Input: dimensioned drawing with shaded views. Units: mm. Origin: part minimum x, y, z. Give positions to 0.01 mm unless a question says otherwise; leave off trailing zeros. Write each loop counter-clockwise with the first axis right and the second up, starting at its lowest first coordinate (ties: lowest second). Pieces come first, ordered by that corner, then holes. Notation, with made-up numbers: (57.5, 14) - (79.5, 14) arc R25 ccw to (79.5, 46) - close; hole circle Ø8 at (35.25, -13.75). An arc over 180 degrees is marked (long way). Answer as a JSON object with one key per item and string values. Group by question number.
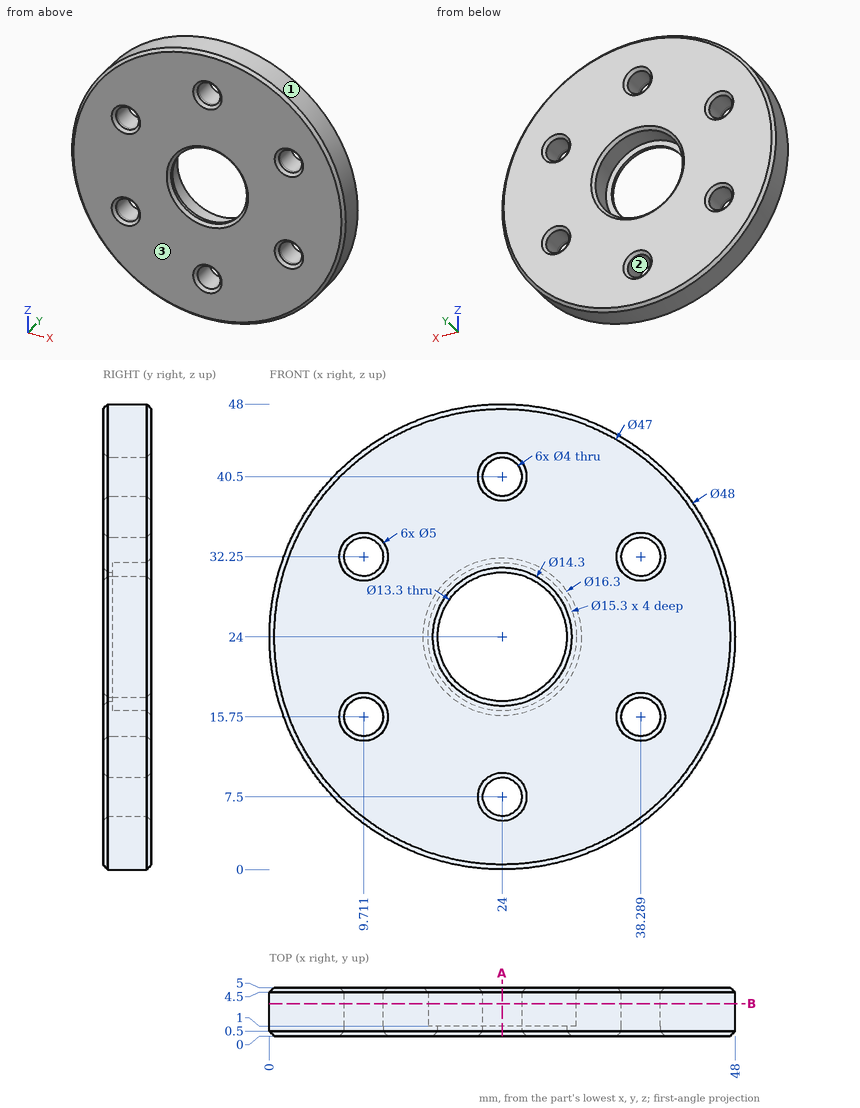
Q1. Section A-A on x = 24. State how many separate pieces and enclosed holes the cut face has.
Q2. Draft query along Z for the marked faces 1, 2 and 3. Return one class per face: released by +Z, released by -Z, zero draft, split by the parting line, or undercut.
Q3. Ray query, probe 1 along Z at (x, y) = (24, 3.1); probe 2 along X at (y, z) = (0.6, 15.75); probe 3 along X at (y, z) = (0.7, 24). Return the intervals inside material, ascending. Write a range as [from, to].
Q4. First-contact query: pin 1 Ø4.5 at (x, z) = (9.71, 32.25) entering from +Y; pin 2 Ø2 at (x, y) = (20.5, 4.5) entering from +Z; pin 3 Ø2 at (x, y) = (23.5, 1) entering from +Z. Flat tips, straight axial feed; report the tip coordinate or a pass-through.
Q5. Section B-B on y = 3.35. Return the cut outline in (x, z).
Taken from the geometry:
{
 "1": {"separate pieces": "4", "enclosed holes": "0"},
 "2": {"face 1": "split by the parting line", "face 2": "undercut", "face 3": "zero draft"},
 "3": {"probe 1": "z = [0, 5.5], [9.5, 16.35], [31.65, 38.5], [42.5, 48]", "probe 2": "x = [1.46, 7.71], [11.71, 36.29], [40.29, 46.54]", "probe 3": "x = [0, 17.35], [30.65, 48]"},
 "4": {"pin 1": "stops at y = 4.75", "pin 2": "stops at z = 47.87", "pin 3": "stops at z = 48"},
 "5": {"outline": "circle Ø48 at (24, 24); hole circle Ø4 at (9.71, 15.75); hole circle Ø4 at (9.71, 32.25); hole circle Ø15.3 at (24, 24); hole circle Ø4 at (24, 7.5); hole circle Ø4 at (24, 40.5); hole circle Ø4 at (38.29, 15.75); hole circle Ø4 at (38.29, 32.25)"}
}
